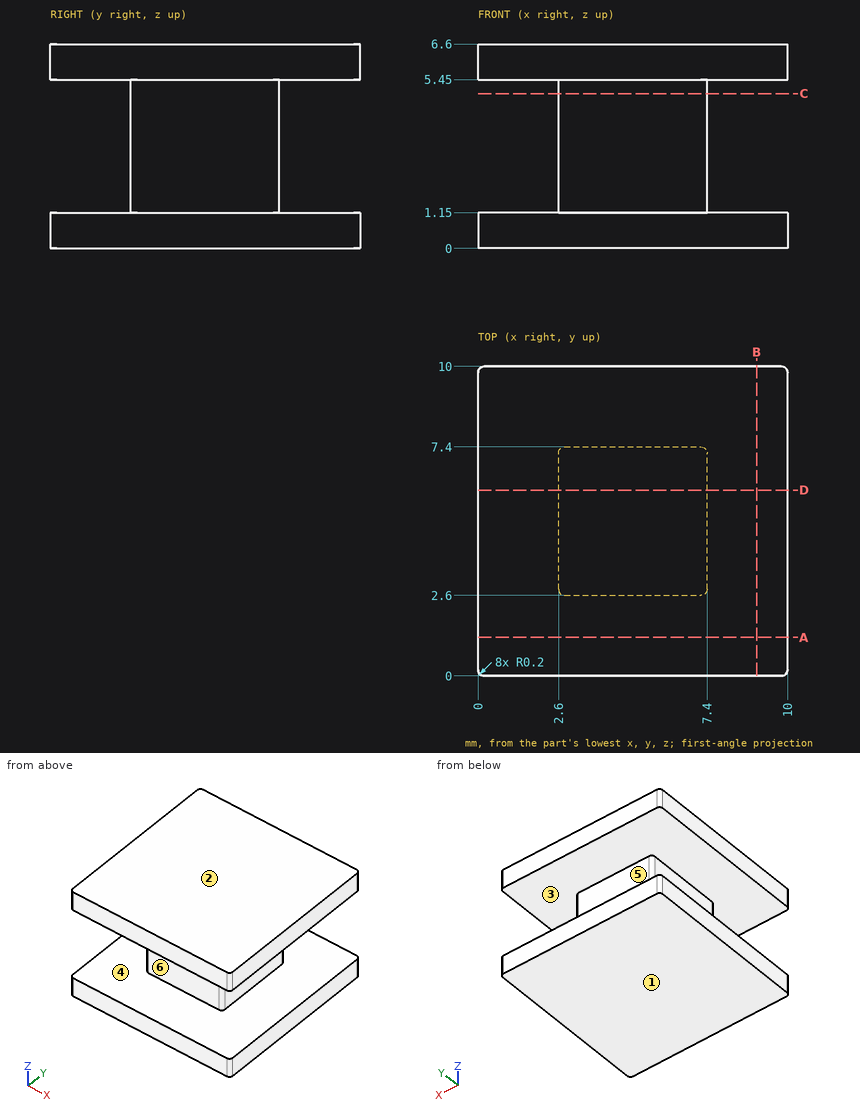
Here's the drawing with two shaded views (mm, measured from the low corner). I have some questions. A direction names the side the tool comes from. Coordinates: 2 decimals unless noted, no trailing zeros. Loops run counter-clockwise (first coordinate to the right, second up) from the corner with the lowest first, then second, coordinate; pieces in that order, holes last.
Item 1: Suppose I cut it at A-A (y = 1.25). Please give me the cut outline in (x, z).
Answers below:
outline: (0, 0) - (10, 0) - (10, 1.15) - (0, 1.15) - close; (0, 5.45) - (10, 5.45) - (10, 6.6) - (0, 6.6) - close
Item 2: Suppose I cut it at C-C (z = 5). Please give me the cut outline in (x, y).
Answers below:
outline: (2.6, 2.8) arc R0.2 ccw to (2.8, 2.6) - (7.2, 2.6) arc R0.2 ccw to (7.4, 2.8) - (7.4, 7.2) arc R0.2 ccw to (7.2, 7.4) - (2.8, 7.4) arc R0.2 ccw to (2.6, 7.2) - close
Item 3: Suppose I cut it at D-D (y = 6). Please give me the cut outline in (x, z), then the cut area to 3 significant figures.
Answers below:
outline: (0, 0) - (10, 0) - (10, 1.15) - (7.4, 1.15) - (7.4, 5.45) - (10, 5.45) - (10, 6.6) - (0, 6.6) - (0, 5.45) - (2.6, 5.45) - (2.6, 1.15) - (0, 1.15) - close
area: 43.6 mm2
Item 4: Which directions (+Z, -Z, +X, -X, +Y, -Y) give clear straight access to the entire face, cutting with the end or side of a thin tool? Please do the marked faces 4, 5 and 6.
Answers below:
face 4: none
face 5: +X, -X, +Y
face 6: +X, -X, -Y
Item 5: Please list where these lines run through material, in increasing order: L1, parallel to Z at x = 5.75, y = 8.5; L2, parallel to Y at x = 7, z = 1.5.
Answers below:
L1: z = 0 to 1.15, 5.45 to 6.6
L2: y = 2.6 to 7.4
Item 6: I'm going to push flat-ended pins straight in: pin 1 (5 mm diameter, centred on x = 6, y = 3.5, fed in from -Z); pin 2 (1 mm diameter, centred on x = 5, z = 4.5, fed in from -Y); pin 3 (2 mm diameter, centred on x = 5, z = 4, fed in from +Y); pin 4 (1.5 mm diameter, centred on y = 3, z = 4.5, fed in from +X). Where does each tip first touch, or does it pass through?
Answers below:
pin 1: stops at z = 0
pin 2: stops at y = 2.6
pin 3: stops at y = 7.4
pin 4: stops at x = 7.4
Item 7: If we mould it in two halves opening along Z, with no side actions, what happens to the marked faces 1, 2 and 3? For each: released by +Z, released by -Z, zero draft, split by the parting line, or undercut.
Answers below:
face 1: released by -Z
face 2: released by +Z
face 3: undercut
